from build123d import *

# Parameters (mm, degrees)
ESQUISSE1_W             = 15
ESQUISSE1_H             = 4
BOSS_EXTRU_1_DEPTH      = 5
ESQUISSE2_W             = 5
ESQUISSE2_H             = 1.8
ENL_V_MAT_EXTRU_1_DEPTH = 5
ESQUISSE3_R             = 1
ENL_V_MAT_EXTRU_2_DEPTH = 5


with BuildPart() as part:
    # Esquisse1 → Boss.-Extru.1 (new body)
    with BuildSketch(Plane(origin=(0, 0, 0), x_dir=(1, 0, 0), z_dir=(0, 1, 0))):
        Rectangle(ESQUISSE1_W, ESQUISSE1_H)
    extrude(amount=BOSS_EXTRU_1_DEPTH)

    # Esquisse2 → Enlèv. mat.-Extru.1 (cut)
    with BuildSketch(Plane(origin=(0, 5, 0), x_dir=(1, 0, 0), z_dir=(0, 1, 0))):
        with Locations((0, 1.1)):
            Rectangle(ESQUISSE2_W, ESQUISSE2_H)
    extrude(amount=-ENL_V_MAT_EXTRU_1_DEPTH, mode=Mode.SUBTRACT)

    # Esquisse3 → Enlèv. mat.-Extru.2 (cut)
    with BuildSketch(Plane(origin=(0, 0, -2), x_dir=(-1, 0, 0), z_dir=(0, 0, -1))):
        with Locations((5, 2.5)):
            Circle(ESQUISSE3_R)
        with Locations((-5, 2.5)):
            Circle(ESQUISSE3_R)
    extrude(amount=-ENL_V_MAT_EXTRU_2_DEPTH, mode=Mode.SUBTRACT)


solid = part.part
The model under review builds one solid part; all positions refer to its coordinate system, in mm. A direction names the side the tool comes from. Round coordinates to 2 decimals unless told otherwise and drop trailing zeros. Order: outer loops, then holes, each group sorted by start corner. A loop starts at its lowest first (then second) coordinate and runs counter-clockwise, first axis right, second up. Notation, with made-up numbers: (18.5, 88.5) -> (64.5, 88.5) arc R26 ccw to (64.5, 126.5) -> close; hole circle Ø8 at (-22, 15.25). An arc over 180 degrees is marked (long way). Write item = value, one per line. Start each with the question number.
Item 1: Consider section C-C on x = -5. Write out the cut boundary in (y, z).
Item 2: For line 1 along Y through (x, z) = (-5, 0.6); line 2 along X through (y, z) = (1.7, -0.95); line 3 along X through (y, z) = (4.45, -0.7), list the stretches that pass through material, from the lowest coordinate up.
Item 3: Consider section A-A on z = -1.7. Write out the cut boundary in (x, y).
Item 4: For faces 4 (the face through (-7.5, 2, 0)), 5 (the face through (-2.5, 3, -1)), list the 3-axis set-ups (+Z, -Z, +X, -X, +Y, -Y) from which the entire face can be reached by the end or side of a thin tool; tool diameter is ignored.
Item 5: Mouldability with a two-part tool opening along Y and no side actions: class faces 1 (the face through (0, 0, 0)), 2 (the face through (-4.87, 3.49, -0.03)), 3 (the face through (7.5, 2, 0)) as released by +Y, released by -Y, zero draft, split by the parting line, or undercut.
Item 6: Consider section D-D on y = 4. Write out the cut boundary in (x, z), plus the area to 3 significant figures.
Item 7: Clearance check with a flat-ended pin moving along its axis: pin 1 Ø1.2 at (x, y) = (-5, 2.5) entering from -Z. State where the tip first meets the part, or that it passes through.
Item 8: Consider section B-B on y = 2.5. Write out the cut boundary in (x, z).
Conclusion:
q1.outline = (0, -2) -> (1.5, -2) -> (1.5, 2) -> (0, 2) -> close; (3.5, -2) -> (5, -2) -> (5, 2) -> (3.5, 2) -> close
q2.line_1 = 0 to 1.5, 3.5 to 5
q2.line_2 = -7.5 to -5.6, -4.4 to -2.5, 2.5 to 4.4, 5.6 to 7.5
q2.line_3 = -7.5 to -2.5, 2.5 to 7.5
q3.outline = (-7.5, 0) -> (-2.5, 0) -> (-2.5, 5) -> (-7.5, 5) -> close; (2.5, 0) -> (7.5, 0) -> (7.5, 5) -> (2.5, 5) -> close; hole circle Ø2 at (-5, 2.5); hole circle Ø2 at (5, 2.5)
q4.face_4 = +Z, -Z, -X, +Y, -Y
q4.face_5 = -Z, +Y, -Y
q5.face_1 = released by -Y
q5.face_2 = undercut
q5.face_3 = zero draft
q6.outline = (-7.5, -2) -> (-2.5, -2) -> (-2.5, -0.2) -> (2.5, -0.2) -> (2.5, -2) -> (7.5, -2) -> (7.5, 2) -> (-7.5, 2) -> close
q6.area = 51.0 mm2
q7.pin_1 = through
q8.outline = (-7.5, -2) -> (-6, -2) -> (-6, 2) -> (-7.5, 2) -> close; (-4, -2) -> (-2.5, -2) -> (-2.5, -0.2) -> (2.5, -0.2) -> (2.5, -2) -> (4, -2) -> (4, 2) -> (-4, 2) -> close; (6, -2) -> (7.5, -2) -> (7.5, 2) -> (6, 2) -> close
